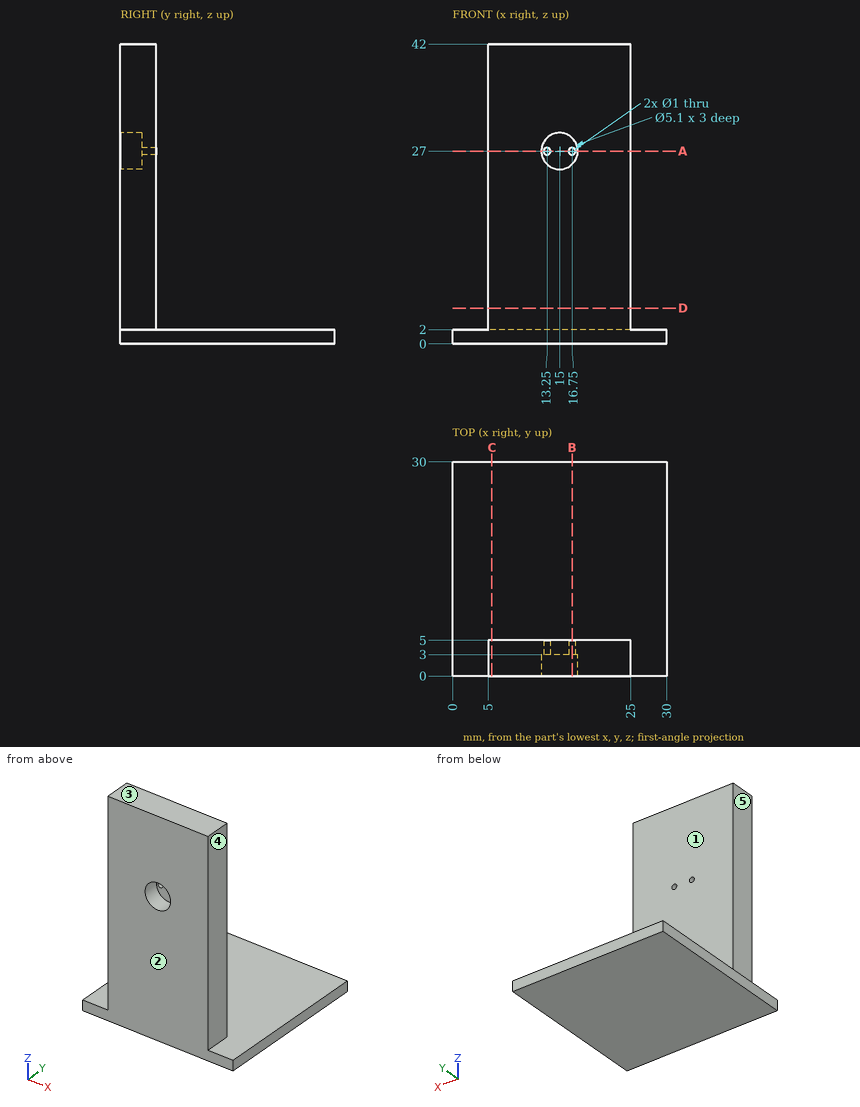
Check sheet for the drawn part. Datum: minimum x, y, z corner. Units: mm. A direction names the side the tool comes from. Coordinates: 2 decimals unless noted, no trailing zeros. Loops run counter-clockwise (first coordinate to the right, second up) from the corner with the lowest first, then second, coordinate; pieces in that order, holes last. Notation, with made-up numbers: M 32,14.5 L 37,14.5 A6 cw 37,23.5 Z; hole C -33.5,-35 d11. An arc over 180 degrees is marked long. Answer as a JSON object with one key per item and string values.
1. Sectioned sample at D-D on z = 5. Record the cut outline in (x, y), and give its area (3 significant figures).
Outcome:
{"outline": "M 5,0 L 25,0 L 25,5 L 5,5 Z", "area": "100 mm²"}
2. Sectioned sample at B-B on x = 16.75. Record the cut outline in (y, z).
Outcome:
{"outline": "M 0,0 L 30,0 L 30,2 L 5,2 L 5,26.5 L 3,26.5 L 3,25.15 L 0,25.15 Z; M 0,28.85 L 3,28.85 L 3,27.5 L 5,27.5 L 5,42 L 0,42 Z"}
3. Depth check by flat-ended pin: P1, Ø1.5, axis at y = 3, z = 31, coming from the +X side; P2, Ø10, axis at y = 10.5, z = 20.5, coming from the -X side; P3, Ø1, axis at x = 14, z = 35, coming from the +Y side; P4, Ø15, axis at x = 16.5, y = 14.5, coming from the +Z side. Enter the tip coordinate at first touch or a pass-through.
Outcome:
{"P1": "x = 25", "P2": "through", "P3": "y = 5", "P4": "z = 2"}
4. Sectioned sample at C-C on x = 5.5. Record the cut outline in (y, z).
Outcome:
{"outline": "M 0,0 L 30,0 L 30,2 L 5,2 L 5,42 L 0,42 Z"}
5. Sectioned sample at A-A on z = 27. Record the cut outline in (x, y).
Outcome:
{"outline": "M 5,0 L 12.45,0 L 12.45,3 L 12.75,3 L 12.75,5 L 5,5 Z; M 13.75,3 L 16.25,3 L 16.25,5 L 13.75,5 Z; M 17.25,3 L 17.55,3 L 17.55,0 L 25,0 L 25,5 L 17.25,5 Z"}
6. Scan lines: L1, parallel to Z at x = 15, y = 1.1; L2, parallel to Z at x = 16.75, y = 3.6; L3, parallel to Z at x = 8.5, y = 20.25. Record each from-to range of solid material in increasing order. Write a range as from..to.
Outcome:
{"L1": "0..24.45, 29.55..42", "L2": "0..26.5, 27.5..42", "L3": "0..2"}
7. Access from +Z, -Z, +X, -X, +Y, -Y to the whole of each face (thin tool, end or side, straight path). Record for the marked faces 1, 2, 3, 4 and 5.
Outcome:
{"face 1": "+Z, +X, -X, +Y", "face 2": "+Z, -Z, +X, -X, -Y", "face 3": "+Z, +X, -X, +Y, -Y", "face 4": "+Z, +X, +Y, -Y", "face 5": "+Z, -X, +Y, -Y"}
